Verification items for the finished model (mm, model axes). Face numbers are marked on the shaded views. Round coordinates to 2 decimals unless told otherwise and drop trailing zeros. Loops run counter-clockwise (first coordinate to the right, second up) from the corner with the lowest first, then second, coordinate; pieces in that order, holes last.
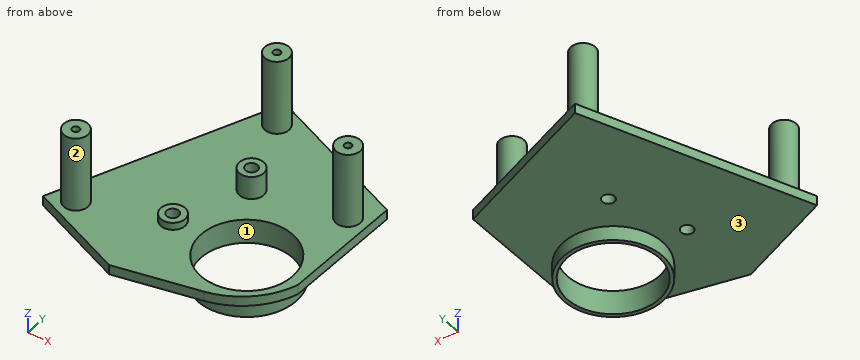
from build123d import *

# Parameters (mm, degrees)
F0_R     = 20.4
F0_R_2   = 18.9
F1_DEPTH = 10
F0_R_3   = 2.5
F2_DEPTH = 4
F3_R     = 5
F3_R_2   = 2.5
F4_DEPTH = 3
F5_DEPTH = 9.5
F3_R_3   = 1.5
F6_DEPTH = 31


with BuildPart() as f1:
    # F0 (on Top) → F1 (new body)
    with BuildSketch(Plane.XY):
        Circle(F0_R)
        Circle(F0_R_2, mode=Mode.SUBTRACT)
    extrude(amount=-F1_DEPTH)

    # F0 (on Top) → F2 (join)
    with BuildSketch(Plane.XY):
        with BuildLine():
            Line((-37.936959, 71.902178), (-73.271744, -15.75))
            Line((-73.271744, -15.75), (-33.738027, -31.68703))
            Line((-33.738027, -31.68703), (0, -23.967391))
            ThreePointArc((0, -23.967391), (14.458763, -16.268714), (23.060463, -2.328261))
            Line((23.060463, -2.328261), (23.060463, 47.312592))
            Line((23.060463, 47.312592), (-37.936959, 71.902178))
        make_face()
        with Locations((-30.9, 0)):
            Circle(F0_R_3, mode=Mode.SUBTRACT)
        Circle(F0_R, mode=Mode.SUBTRACT)
        with Locations((-19.540395, 28.736203)):
            Circle(F0_R_3, mode=Mode.SUBTRACT)
    extrude(amount=-F2_DEPTH)

    # F3 (on face) → F4 (join)
    with BuildSketch(Plane.XY):
        with Locations((-30.81522, 0)):
            Circle(F3_R)
        with Locations((-30.9, 0)):
            Circle(F3_R_2, mode=Mode.SUBTRACT)
    extrude(amount=F4_DEPTH)

    # F3 (on face) → F5 (join)
    with BuildSketch(Plane.XY):
        with Locations((-19.565957, 28.747549)):
            Circle(F3_R)
        with Locations((-19.540395, 28.736203)):
            Circle(F3_R_2, mode=Mode.SUBTRACT)
    extrude(amount=F5_DEPTH)

    # F3 (on face) → F6 (join)
    with BuildSketch(Plane.XY):
        with Locations((15.060463, 36.312592)):
            Circle(F3_R)
        with Locations((15.060463, 36.312592)):
            Circle(F3_R_3, mode=Mode.SUBTRACT)
        with Locations((-33.508272, 61.491284)):
            Circle(F3_R)
        with Locations((-33.508272, 61.491284)):
            Circle(F3_R_3, mode=Mode.SUBTRACT)
        with Locations((-62.860849, -11.321312)):
            Circle(F3_R)
        with Locations((-62.860849, -11.321312)):
            Circle(F3_R_3, mode=Mode.SUBTRACT)
    extrude(amount=F6_DEPTH)


solid = f1.part
1. Scan lines: L1, parallel to Y at x = 0, z = -7; L2, parallel to Z at x = 15.5, y = 47.5; L3, parallel to Y at x = 0, z = -3.5. Record each from-to range of solid material in increasing order.
2. Gauge pin test, flat ends, axial feed: P1, Ø1.5, axis at x = 15.5, y = 36.5, coming from the +Z side; P2, Ø8, axis at x = -22, y = 22, coming from the -Z side; P3, Ø8, axis at x = -18.5, y = 30.5, coming from the +Z side. Record the tip position at first contact, or that the pin passes through.
3. Release check for a two-part mould opening along Y. For the marked faces 1, 2 and 3 record: released by +Y, released by -Y, zero draft, split by the parting line, or undercut.
4. Section check A-A (x = 15). Enter the section's corners in (y, z), then the cut area to 3 significant figures.
5. Section check B-B (z = 18). Enter the section's corners in (x, y).
6. Section check C-C (y = 0). Enter the section's corners in (x, z), then the cut area to 3 significant figures.
7. Section check D-D (z = -2). Enter the section's corners in (x, y), then the cut area to 3 significant figures.
Taken from the geometry:
1. L1: y = -20.4 to -18.9, 18.9 to 20.4
1. L2: z = -4 to 0
1. L3: y = -23.97 to -18.9, 18.9 to 56.61
2. P1: stops at z = 0
2. P2: stops at z = -4
2. P3: stops at z = 9.5
3. face 1: undercut
3. face 2: split by the parting line
3. face 3: zero draft
4. outline: (-15.75, -4) - (-13.83, -4) - (-13.83, -10) - (-11.5, -10) - (-11.5, 0) - (-15.75, 0) - close; (11.5, -10) - (13.83, -10) - (13.83, -4) - (50.56, -4) - (50.56, 0) - (41.31, 0) - (41.31, 31) - (37.81, 31) - (37.81, 0) - (34.81, 0) - (34.81, 31) - (31.31, 31) - (31.31, 0) - (11.5, 0) - close
4. area: 418 mm2
5. outline: circle Ø10 at (-62.86, -11.32); circle Ø10 at (-33.51, 61.49); circle Ø10 at (15.06, 36.31); hole circle Ø3 at (-62.86, -11.32); hole circle Ø3 at (-33.51, 61.49); hole circle Ø3 at (15.06, 36.31)
6. outline: (-66.92, -4) - (-33.4, -4) - (-33.4, 3) - (-35.82, 3) - (-35.82, 0) - (-66.92, 0) - close; (-28.4, -4) - (-20.4, -4) - (-20.4, -10) - (-18.9, -10) - (-18.9, 0) - (-25.82, 0) - (-25.82, 3) - (-28.4, 3) - close; (18.9, -10) - (20.4, -10) - (20.4, -4) - (23.06, -4) - (23.06, 0) - (18.9, 0) - close
6. area: 222 mm2
7. outline: (-73.27, -15.75) - (-33.74, -31.69) - (0, -23.97) arc R31.35 ccw to (23.06, -2.33) - (23.06, 47.31) - (-37.94, 71.9) - close; hole circle Ø5 at (-30.9, 0); hole circle Ø5 at (-19.54, 28.74); hole circle Ø37.8 at (0, 0)
7. area: 5,740 mm2
